The listing builds one solid part. Answer for the finished solid, in the listing's coordinates (mm). A direction names the side the tool comes from. Round coordinates to 2 decimals unless told otherwise and drop trailing zeros. Loops run counter-clockwise (first coordinate to the right, second up) from the corner with the lowest first, then second, coordinate; pieces in that order, holes last. Notation, with made-up numbers: M 83,-37 L 127,-37 A30 cw 127,1 Z; hole C -29,15.5 d11. An arc over 180 degrees is marked long. Put each result on its own line as item: value. Start each with the question number.
(1) Which of the six approach directions +Z, -Z, +X, -X, +Y, -Y give full straight-line access (tool end or side, diameter ignored) to faces 1 (the face through (127, 0, -18)), 2 (the face through (39.49, -0.07, 139.05))?
(2) Straight lines are drawn through the part: line 1 (Z direction, x = 2, y = -2); line 2 (X direction, y = 1.25, z = 116); line 3 (Z direction, x = 59.5, y = -4). For each, find the intervals that lie inside material, in ascending order.
(3) Section C-C, the plane y = 2.5 is taken. Count the separate pieces of the cut face and the enclosed holes in it, then the cut area to 3 significant figures.
(4) Section D-D, the plane x = 76 is taken. Determine the outline of the cut face in (y, z).
(5) Section B-B, the plane x = -18 is taken. Determine the outline of the cut face in (y, z), then the cut area to 3 significant figures.
(6) Determine the mould class of faces 3 (the face through (-2, 0, -165.1)), 4 (the face through (1.48, -0.07, 165.097)), 5 (the face through (-39.65, -0.07, 124.91)) for opening direction Z: released by +Z, released by -Z, zero draft, split by the parting line, or undercut.
(7) Flat-ended cylindrical pins translate along their axes: P1, Ø4, axis at x = 89.75, z = 29.75, coming from the -Y side; P2, Ø1.5, axis at x = -92.5, y = -2, coming from the +Z side; P3, Ø1, axis at x = -99.5, y = 0, coming from the +Z side. Find the tip coordinate at first contact, or state that the pin passes through.
(8) Section A-A, the plane z = 137 is taken. Determine the outline of the cut face in (x, y), then the cut area to 3 significant figures.
```python
from build123d import *

# Parameters (mm, degrees)
F0_R     = 2.25
F0_R_2   = 2.125
F0_W     = 85
F0_H     = 20
F1_DEPTH = 5
F2_R     = 9.99999
F3_R     = 30


# Not quite as in the source:
# - a fillet or chamfer is up to 0.001 mm smaller than in the source, because OpenCascade refuses the exact size


with BuildPart() as f1:
    # F0 (on Front) → F1 (new body, symmetric)
    with BuildSketch(Plane.XZ):
        with BuildLine():
            Line((-127, -165.1), (127, -165.1))
            Line((127, -165.1), (127, 145.1))
            ThreePointArc((127, 145.1), (0, 165.1), (-127, 145.1))
            Line((-127, 145.1), (-127, -165.1))
        make_face()
        with Locations((-92, -34.75)):
            Circle(F0_R, mode=Mode.SUBTRACT)
        with Locations((-77, -34.75)):
            Circle(F0_R, mode=Mode.SUBTRACT)
        with Locations((-84.5, 0)):
            Circle(F0_R, mode=Mode.SUBTRACT)
        with Locations((2, -140.1)):
            Circle(F0_R, mode=Mode.SUBTRACT)
        with Locations((2, -130.1)):
            Circle(F0_R, mode=Mode.SUBTRACT)
        with Locations((59.5, -135.1)):
            Circle(F0_R, mode=Mode.SUBTRACT)
        with Locations((117, -140.1)):
            Circle(F0_R, mode=Mode.SUBTRACT)
        with Locations((117, -130.1)):
            Circle(F0_R, mode=Mode.SUBTRACT)
        with Locations((8, -34.75)):
            Circle(F0_R, mode=Mode.SUBTRACT)
        with Locations((23, -34.75)):
            Circle(F0_R, mode=Mode.SUBTRACT)
        with Locations((11, -15.5)):
            Circle(F0_R_2, mode=Mode.SUBTRACT)
        with BuildLine():
            ThreePointArc((13.5482954545, -1.1195308693), (13.25, 0), (13.5482954545, 1.1195308693))
            ThreePointArc((13.5482954545, 1.1195308693), (27.0602860471, 12.9879205243), (39.5, 0))
            ThreePointArc((39.5, 0), (27.0602860471, -12.9879205243), (13.5482954545, -1.1195308693))
        make_face(mode=Mode.SUBTRACT)
        with Locations((42, -15.5)):
            Circle(F0_R_2, mode=Mode.SUBTRACT)
        with Locations((89.75, -29.75)):
            Circle(F0_R, mode=Mode.SUBTRACT)
        with Locations((84.5, 0)):
            Circle(F0_R, mode=Mode.SUBTRACT)
        with Locations((107, -27)):
            Circle(F0_R, mode=Mode.SUBTRACT)
        with Locations((119.5, 0)):
            Circle(F0_R, mode=Mode.SUBTRACT)
        with Locations((-92, 34.75)):
            Circle(F0_R, mode=Mode.SUBTRACT)
        with Locations((-77, 34.75)):
            Circle(F0_R, mode=Mode.SUBTRACT)
        with Locations((11, 15.5)):
            Circle(F0_R_2, mode=Mode.SUBTRACT)
        with Locations((8, 34.75)):
            Circle(F0_R, mode=Mode.SUBTRACT)
        with Locations((23, 34.75)):
            Circle(F0_R, mode=Mode.SUBTRACT)
        with Locations((42, 15.5)):
            Circle(F0_R_2, mode=Mode.SUBTRACT)
        with Locations((89.75, 29.75)):
            Circle(F0_R, mode=Mode.SUBTRACT)
        with Locations((107, 27)):
            Circle(F0_R, mode=Mode.SUBTRACT)
        with Locations((2, 114.9)):
            Circle(F0_R, mode=Mode.SUBTRACT)
        with Locations((59.5, 119.9)):
            Circle(F0_R, mode=Mode.SUBTRACT)
        with Locations((0, 131.9)):
            Rectangle(F0_W, F0_H, mode=Mode.SUBTRACT)
        with Locations((117, 114.9)):
            Circle(F0_R, mode=Mode.SUBTRACT)
        with Locations((117, 124.9)):
            Circle(F0_R, mode=Mode.SUBTRACT)
    extrude(amount=F1_DEPTH, both=True)

    # F2 (radius 10 in the source; OpenCascade refuses exactly that, so slightly less here)
    f2_edges = [f1.edges().sort_by_distance(p)[0] for p in [
        (-127, 0, -165.1),
        (127, 0, -165.1),
        (-42.5, 0, 141.9),
        (-42.5, 0, 121.9),
        (42.5, 0, 141.9),
        (42.5, 0, 121.9),
    ]]
    fillet(f2_edges, radius=F2_R)

    # F3
    f3_edges = [f1.edges().sort_by_distance(p)[0] for p in [
        (127, 0, 145.1),
        (-127, 0, 145.1),
    ]]
    fillet(f3_edges, radius=F3_R)


solid = f1.part
```
Recorded:
1. face 1: +Z, -Z, +X, +Y, -Y
1. face 2: +Y, -Y
2. line 1: z = -165.1 to -142.35, -137.85 to -132.35, -127.85 to 112.65, 117.15 to 121.9, 141.9 to 165.1
2. line 2: x = -127 to 0.04, 3.96 to 115.04, 118.96 to 127
2. line 3: z = -165.1 to -137.35, -132.85 to 117.65, 122.15 to 160.79
3. separate pieces: 1
3. enclosed holes: 30
3. area: 79,400 mm²
4. outline: M -5,-165.1 L 5,-165.1 L 5,158.05 L -5,158.05 Z
5. outline: M -5,-165.1 L 5,-165.1 L 5,121.9 L -5,121.9 Z; M -5,141.9 L 5,141.9 L 5,164.71 L -5,164.71 Z
5. area: 3,100 mm²
6. face 3: released by -Z
6. face 4: released by +Z
6. face 5: undercut
7. P1: passes through
7. P2: stops at z = 154.79
7. P3: stops at z = 153.07
8. outline: M -123.33,-5 L -41.1,-5 L -41.1,5 L -123.33,5 Z; M 41.1,-5 L 123.33,-5 L 123.33,5 L 41.1,5 Z
8. area: 1,640 mm²
